Check sheet for the modelled part. Datum: model origin and axes. Units: mm. Face numbers are marked on the shaded views. A direction names the side the tool comes from. Round coordinates to 2 decimals unless told otherwise and drop trailing zeros. Order: outer loops, then holes, each group sorted by start corner. A loop starts at its lowest first (then second) coordinate and runs counter-clockwise, first axis right, second up. Notation, with made-up numbers: (57.25, -7.5) -> (88.25, -7.5) arc R24 cw to (88.25, 30.5) -> close; hole circle Ø1 at (85.25, 77.25). An arc over 180 degrees is marked (long way). Answer in a Markdown table with one row per item. Add a question column.
1. Access from +Z, -Z, +X, -X, +Y, -Y to the whole of each face (thin tool, end or side, straight path). Record for the marked faces 1 and 2.
2. Material ranges on L1, parallel to X at y = -11, z = -13; L2, parallel to Y at x = -48, z = 0.5; L3, parallel to X at y = -2.5, z = -2, recorded low to high. Write a range as from..to.
3. Sectioned sample at A-A, the plane y = 0. Record the boundary of the cut face in (x, z), then the cut area to 3 significant figures.
4. Sectioned sample at D-D, the plane z = -7. Record the boundary of the cut face in (x, y), then the cut area to 3 significant figures.
5. Depth check by flat-ended pin: P1, Ø2, axis at x = -13.5, z = -3.5, coming from the +Y side; P2, Ø10, axis at x = -2, y = 12, coming from the -Z side; P3, Ø18.5, axis at y = -7, z = -7, coming from the +X side; P4, Ø4, axis at x = -32.5, y = -12, coming from the +Z side. Enter the tip coordinate at first touch or a pass-through.
6. Sectioned sample at C-C, the plane x = 1. Record the boundary of the cut face in (y, z), then the cut area to 3 significant figures.
7. Sectioned sample at B-B, the plane z = -2. Record the boundary of the cut face in (x, y), then the cut area to 3 significant figures.
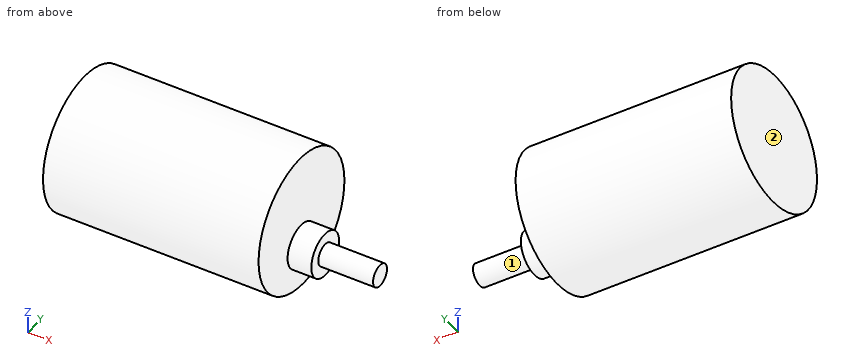
```python
from build123d import *

# Parameters (mm, degrees)
F0_R     = 18.5
F1_DEPTH = 59
F2_R     = 6
F3_DEPTH = 6.5
F4_R     = 3
F5_DEPTH = 15


with BuildPart() as f1:
    # F0 (on Right) → F1 (new body)
    with BuildSketch(Plane.YZ):
        Circle(F0_R)
    extrude(amount=-F1_DEPTH)

    # F2 (on face) → F3 (join)
    with BuildSketch(Plane.YZ):
        with Locations((0, -7)):
            Circle(F2_R)
    extrude(amount=F3_DEPTH)

    # F4 (on face) → F5 (join)
    with BuildSketch(Plane.YZ.offset(6.5)):
        with Locations((0, -7)):
            Circle(F4_R)
    extrude(amount=F5_DEPTH)


solid = f1.part
```
Answer key:
| question | item | result |
|---|---|---|
| 1 | face 1 | +X |
| 1 | face 2 | +Z, -Z, -X, +Y, -Y |
| 2 | L1 | x = -59..0 |
| 2 | L2 | y = -18.49..18.49 |
| 2 | L3 | x = -59..6.5 |
| 3 | outline | (-59, -18.5) -> (0, -18.5) -> (0, -13) -> (6.5, -13) -> (6.5, -10) -> (21.5, -10) -> (21.5, -4) -> (6.5, -4) -> (6.5, -1) -> (0, -1) -> (0, 18.5) -> (-59, 18.5) -> close |
| 3 | area | 2,350 mm² |
| 4 | outline | (-59, -17.12) -> (0, -17.12) -> (0, -6) -> (6.5, -6) -> (6.5, -3) -> (21.5, -3) -> (21.5, 3) -> (6.5, 3) -> (6.5, 6) -> (0, 6) -> (0, 17.12) -> (-59, 17.12) -> close |
| 4 | area | 2,190 mm² |
| 5 | P1 | stops at y = 18.33 |
| 5 | P2 | stops at z = -17.12 |
| 5 | P3 | stops at x = 21.5 |
| 5 | P4 | stops at z = 15.56 |
| 6 | outline | circle Ø12 at (0, -7) |
| 6 | area | 113 mm² |
| 7 | outline | (-59, -18.39) -> (0, -18.39) -> (0, -3.32) -> (6.5, -3.32) -> (6.5, 3.32) -> (0, 3.32) -> (0, 18.39) -> (-59, 18.39) -> close |
| 7 | area | 2,210 mm² |
